Answer from the drawing. Dimensions are ordinates in mm from the lowest x, y and z of the part. A direction names the side the tool comes from. Coordinates: 2 decimals unless noted, no trailing zeros. Loops run counter-clockwise (first coordinate to the right, second up) from the corner with the lowest first, then second, coordinate; pieces in that order, holes last. Notation, with made-up numbers: (26.25, 68) - (75.25, 68) arc R34 cw to (75.25, 102) - close; hole circle Ø10 at (77, 53.5). An arc over 180 degrees is marked (long way). One line per question, with ' | ' between items. Start each with the question number.
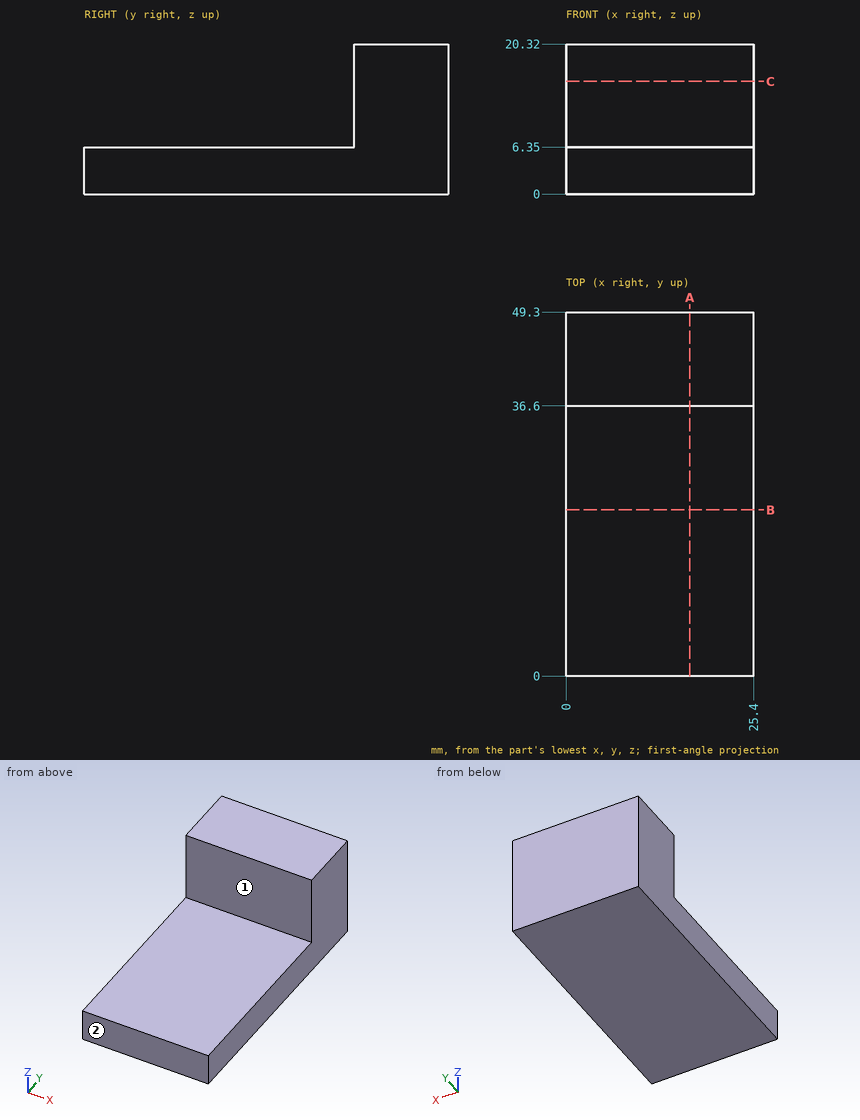
1) Given pin 1 Ø1.5 at (x, y) = (4, 28.5) entering from +Z; pin 2 Ø8 at (x, z) = (21.5, 11.5) entering from -Y, each flat-ended and moving along its own axis, determine where each tip first touches the part or whether it passes through.
2) Which of the six approach directions +Z, -Z, +X, -X, +Y, -Y give full straight-line access (tool end or side, diameter ignored) to the marked faces 1 and 2?
3) The part is cut by section A-A on x = 16.75. Write down the section's boundary in (y, z).
4) Find the intervals of material crossed by line 1 along Y through (x, z) = (16.5, 11.5); line 2 along Z through (x, y) = (15.5, 22.5), in increasing order. Write a range as from..to.
5) The part is cut by section C-C on z = 15.25. Write down the section's boundary in (x, y), and give its area (3 significant figures).
6) The part is cut by section B-B on y = 22.5. Write down the section's boundary in (x, z), and give its area (3 significant figures).
Answer below:
1) pin 1: z = 6.35 | pin 2: y = 36.6
2) face 1: +Z, +X, -X, -Y | face 2: +Z, -Z, +X, -X, -Y
3) outline: (0, 0) - (49.3, 0) - (49.3, 20.32) - (36.6, 20.32) - (36.6, 6.35) - (0, 6.35) - close
4) line 1: 36.6..49.3 | line 2: 0..6.35
5) outline: (0, 36.6) - (25.4, 36.6) - (25.4, 49.3) - (0, 49.3) - close | area: 323 mm2
6) outline: (0, 0) - (25.4, 0) - (25.4, 6.35) - (0, 6.35) - close | area: 161 mm2
